```python
from build123d import *

# Parameters (mm, degrees)
F0_R     = 41.7000635609
F1_DEPTH = 25.4
F2_R     = 21.0958969827
F3_DEPTH = 5.08


# Not quite as in the source:
# - a fillet or chamfer that OpenCascade refuses, or shapes differently, is made with other operations: its cross-section is extruded or revolved along the edge and cut away or added


with BuildPart() as f1:
    # F0 (on Top) → F1 (new body)
    with BuildSketch(Plane.XY):
        Circle(F0_R)
    extrude(amount=-F1_DEPTH)

    # F2 (on face) → F3 (cut)
    with BuildSketch(Plane.XY):
        Circle(F2_R)
    extrude(amount=-F3_DEPTH, mode=Mode.SUBTRACT)

    # F4: fillet of radius 7.62 on 1 edges, made by hand

    # F4_s1 → F4_t2 (revolve)
    with BuildSketch(Plane.XZ):
        with BuildLine():
            ThreePointArc((21.0958969827, 0), (18.3111011371, -3.6817039467), (13.9116920859, -5.08))
            Line((13.9116920859, -5.08), (21.0958969827, -5.08))
            Line((21.0958969827, -5.08), (21.0958969827, 0))
        make_face()
    revolve(axis=Axis((0, 0, -5.08), (0, 0, 1)))


solid = f1.part
```
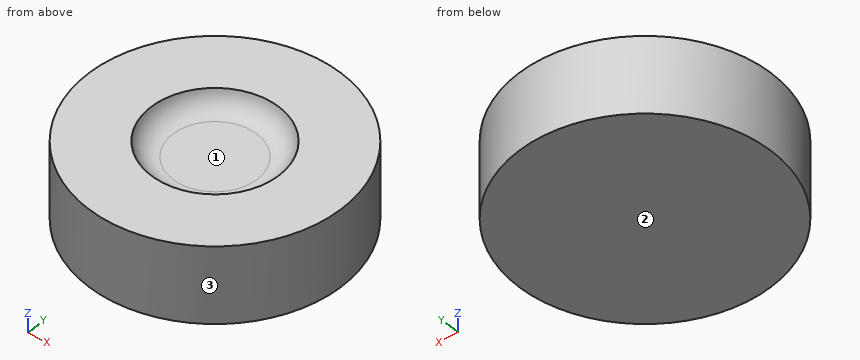
Source: CAD feature listing. Evaluate the final solid. Frame: model axes, mm. Face numbers are marked on the shaded views. Coordinates: 2 decimals unless noted, no trailing zeros. Write each loop counter-clockwise with the first axis right and the second up, starting at its lowest first coordinate (ties: lowest second). Pieces come first, ordered by that corner, then holes. Notation, with made-up numbers: (-0.75, -22.5) -> (54.25, -22.5) arc R17 cw to (54.25, -4.5) -> close; hole circle Ø9 at (56, 9.5). An arc over 180 degrees is marked (long way). Return JSON: item names as keys, results as strings. Group by question number.
1) Section query D-D, the plane z = -3.25. Return loops of the section in (x, y), plus the area to 3 significant figures.
2) Section query C-C, the plane z = -21.75. Return loops of the section in (x, y).
3) Section query A-A, the plane y = 0. Return loops of the section in (x, z), plus the area to 3 significant figures.
4) Mould query, pull axis X, two halves, no side actions, for the marked faces 1, 2 and 3. Classes: +X half, -X half, draft (parallel to the pull), parting line (faces both ways), or undercut.
5) Ray query, line 1 along Z through (x, y) = (4.5, 12); line 2 along Y through (x, z) = (20, -5.25); line 3 along Y through (x, z) = (-12, -3.25). Return the intervals inside material, ascending.
6) Contact query for flat-ended pins moving along their axis: P1, Ø12, axis at x = 2, z = -11.5, coming from the -Y side; P2, Ø2, axis at x = 29.5, z = -20, coming from the -Y side; P3, Ø5, axis at x = -23, z = -12.5, coming from the +Y side. Output: stop coordinate, or through.
From the geometry:
{
 "1": {"outline": "circle Ø83.4 at (0, 0); hole circle Ø37.73 at (0, 0)", "area": "4,340 mm²"},
 "2": {"outline": "circle Ø83.4 at (0, 0)"},
 "3": {"outline": "(-41.7, -25.4) -> (41.7, -25.4) -> (41.7, 0) -> (21.1, 0) arc R7.62 cw to (13.91, -5.08) -> (-13.91, -5.08) arc R7.62 cw to (-21.1, 0) -> (-41.7, 0) -> close", "area": "1,920 mm²"},
 "4": {"face 1": "undercut", "face 2": "draft", "face 3": "parting line"},
 "5": {"line 1": "-25.4 to -5.08", "line 2": "-36.59 to 36.59", "line 3": "-39.94 to -14.56, 14.56 to 39.94"},
 "6": {"P1": "y = -41.7", "P2": "y = -30.44", "P3": "y = 36.31"}
}
